Input: part model. Units: mm. Frame: model coordinates. Face numbers are marked on the shaded views. A direction names the side the tool comes from. Give positions to 0.01 mm unless a question says otherwise; leave off trailing zeros. Loops run counter-clockwise (first coordinate to the right, second up) from the corner with the lowest first, then second, coordinate; pieces in that order, holes last.
from build123d import *

# Parameters (mm, degrees)
F0_R     = 11
F1_DEPTH = 32
F2_R     = 1.5
F3_DEPTH = 5
F5_DEPTH = 32
F6_R     = 3
F7_DEPTH = 17.3
F9_DEPTH = 12


with BuildPart() as f1:
    # F0 (on Front) → F1 (new body)
    with BuildSketch(Plane.XZ):
        Circle(F0_R)
    extrude(amount=F1_DEPTH)

    # F2 (on face) → F3 (cut)
    with BuildSketch(Plane.XZ.offset(32)):
        with Locations((0, 8.5)):
            Circle(F2_R)
        with Locations((-7.361216, -4.25)):
            Circle(F2_R)
        with Locations((7.361216, -4.25)):
            Circle(F2_R)
    extrude(amount=-F3_DEPTH, mode=Mode.SUBTRACT)

    # F4 (on face) → F5 (join)
    with BuildSketch(Plane(origin=(0, 0, 0), x_dir=(-1, 0, 0), z_dir=(0, 1, 0))):
        with BuildLine():
            Line((6.670832, 7.65), (-6.670832, 7.65))
            ThreePointArc((-6.670832, 7.65), (-10.15, 0), (-6.670832, -7.65))
            Line((-6.670832, -7.65), (6.670832, -7.65))
            ThreePointArc((6.670832, -7.65), (10.15, 0), (6.670832, 7.65))
        make_face()
    extrude(amount=F5_DEPTH)

    # F6 (on face) → F7 (join)
    with BuildSketch(Plane.XZ.offset(32)):
        Circle(F6_R)
    extrude(amount=F7_DEPTH)

    # F8 (on face) → F9 (cut)
    with BuildSketch(Plane.XZ.offset(49.3)):
        with BuildLine():
            ThreePointArc((1.658312, 2.5), (0, 3), (-1.658312, 2.5))
            Line((-1.658312, 2.5), (1.658312, 2.5))
        make_face()
    extrude(amount=-F9_DEPTH, mode=Mode.SUBTRACT)


solid = f1.part
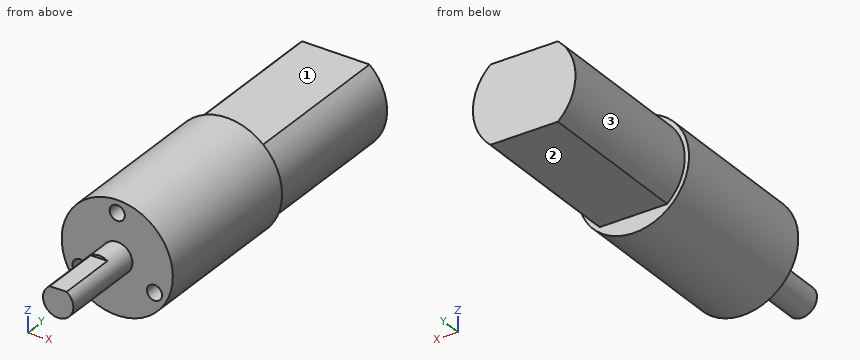
(1) Cut plane B-B (z = 0). Return the cut outline in (x, y), and give its area (3 significant figures).
Values follow:
outline: (-11, -32) - (-3, -32) - (-3, -49.3) - (3, -49.3) - (3, -32) - (11, -32) - (11, 0) - (10.15, 0) - (10.15, 32) - (-10.15, 32) - (-10.15, 0) - (-11, 0) - close
area: 1,460 mm2
(2) Cut plane A-A (x = 0). Return the cut outline in (y, z).
Values follow:
outline: (-49.3, -3) - (-32, -3) - (-32, -11) - (0, -11) - (0, -7.65) - (32, -7.65) - (32, 7.65) - (0, 7.65) - (0, 11) - (-32, 11) - (-32, 10) - (-27, 10) - (-27, 7) - (-32, 7) - (-32, 3) - (-37.3, 3) - (-37.3, 2.5) - (-49.3, 2.5) - close
(3) Cut plane D-D (z = -4.25). Return the cut outline in (x, y).
Values follow:
outline: (-10.15, -32) - (-8.86, -32) - (-8.86, -27) - (-5.86, -27) - (-5.86, -32) - (5.86, -32) - (5.86, -27) - (8.86, -27) - (8.86, -32) - (10.15, -32) - (10.15, 0) - (9.22, 0) - (9.22, 32) - (-9.22, 32) - (-9.22, 0) - (-10.15, 0) - close
(4) Reachability of the marked faces 1, 2 and 3 from +Z, -Z, +X, -X, +Y, -Y: full face, straight path, thin tool, end or side. Return the list, or none.
Values follow:
face 1: +Z, +X, -X, +Y
face 2: -Z, +X, -X, +Y
face 3: -X, +Y
(5) Pin query (flat end, axial travel): pin 1 Ø1 at (x, z) = (-7, -6) entering from -Y; pin 2 Ø1 at (x, y) = (-8, 0) entering from +Z; pin 3 Ø0.9 at (x, z) = (7, -5) entering from -Y. Return the tip coordinate at first contact, or that it passes through.
Values follow:
pin 1: stops at y = -32
pin 2: stops at z = 8.05
pin 3: stops at y = -27
(6) Cut plane C-C (y = -18). Return the cut outline in (x, z).
Values follow:
outline: circle Ø22 at (0, 0)
(7) Ray query, probe 1 along Y at (x, z) = (7, 8); probe 2 along Z at (x, y) = (-8.75, -22.5); probe 3 along Z at (x, y) = (5.5, 6). Return the intervals inside material, ascending.
Values follow:
probe 1: y = -32 to 0
probe 2: z = -6.67 to 6.67
probe 3: z = -7.65 to 7.65
